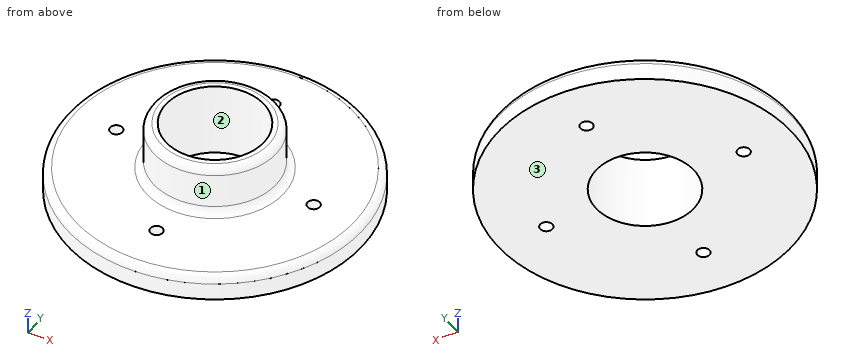
```python
from build123d import *

# Parameters (mm, degrees)
F0_R     = 76.2
F0_R_2   = 25.4
F1_DEPTH = 12.7
F2_R     = 31.75
F2_R_2   = 25.4
F3_DEPTH = 38.1
F4_R     = 3.175
F5_DEPTH = 12.701
F6_R     = 3.81


with BuildPart() as f1:
    # F0 (on Top) → F1 (new body)
    with BuildSketch(Plane.XY):
        Circle(F0_R)
        Circle(F0_R_2, mode=Mode.SUBTRACT)
    extrude(amount=F1_DEPTH)

    # F2 (on Top) → F3 (join)
    with BuildSketch(Plane.XY):
        Circle(F2_R)
        Circle(F2_R_2, mode=Mode.SUBTRACT)
    extrude(amount=F3_DEPTH)

    # F4 (on face) → F5 (cut, through all)
    with BuildSketch(Plane.XY.offset(12.7)):
        with Locations((-50.8, 0)):
            Circle(F4_R)
        with Locations((0, -50.8)):
            Circle(F4_R)
        with Locations((50.8, 0)):
            Circle(F4_R)
        with Locations((0, 50.8)):
            Circle(F4_R)
    extrude(amount=-F5_DEPTH, mode=Mode.SUBTRACT)

    # F6
    f6_edges = [f1.edges().sort_by_distance(p)[0] for p in [
        (-76.2, 0, 12.7),
        (-31.75, 0, 38.1),
        (-31.75, 0, 12.7),
    ]]
    fillet(f6_edges, radius=F6_R)


solid = f1.part
```
CAD build for the part. Positions are in the model's coordinates, mm. Face numbers are marked on the shaded views. Coordinates: 2 decimals unless noted, no trailing zeros. Write each loop counter-clockwise with the first axis right and the second up, starting at its lowest first coordinate (ties: lowest second). Pieces come first, ordered by that corner, then holes. Notation, with made-up numbers: (72, 64) -> (126, 64) arc R30 cw to (126, 86) -> close; hole circle Ø6 at (0, 80). An arc over 180 degrees is marked (long way). Return JSON: item names as keys, results as strings. Group by question number.
Q1. Cut at A-A, the plane y = 0. Give the cut face in (x, z) (3 decimals), then the cut area to 3 significant figures.
Q2. Flat gauge pins, fed straight in: pin 1 (5 mm diameter, centred on x = 14.5, z = 33, fed in from -Y); pin 2 (3 mm diameter, centred on x = -50.5, y = -45, fed in from +Z); pin 3 (2 mm diameter, centred on y = -19.5, z = 23.5, fed in from +X); pin 4 (3 mm diameter, centred on x = 53, y = -42.5, fed in from -Z). Where does each tip first touch, or does it go through?
Q3. Cut at C-C, the plane z = 5. Give the cut face in (x, y) (3 decimals), then the cut area to 3 significant figures.
Q4. Pull direction Y, two halves, no side cores. Call the marked faces 1, 2 and 3: released by +Y, released by -Y, zero draft, split by the parting line, or undercut.
Q5. Drill centre lines: line 1 (Y direction, x = 0, z = 4.5) (3 decimals); line 2 (Y direction, x = 0, z = 24); line 3 (Z direction, x = -37, y = 45). Where is each one in solid material? Low to high.
Q6. Cut at D-D, the plane z = 25.5. Give the cut face in (x, y), then the cut area to 3 significant figures.
Returned:
{
 "1": {"outline": "(-76.2, 0) -> (-53.975, 0) -> (-53.975, 12.7) -> (-72.39, 12.7) arc R3.81 ccw to (-76.2, 8.89) -> close; (-47.625, 0) -> (-25.4, 0) -> (-25.4, 38.1) -> (-27.94, 38.1) arc R3.81 ccw to (-31.75, 34.29) -> (-31.75, 16.51) arc R3.81 cw to (-35.56, 12.7) -> (-47.625, 12.7) -> close; (25.4, 0) -> (47.625, 0) -> (47.625, 12.7) -> (35.56, 12.7) arc R3.81 cw to (31.75, 16.51) -> (31.75, 34.29) arc R3.81 ccw to (27.94, 38.1) -> (25.4, 38.1) -> close; (53.975, 0) -> (76.2, 0) -> (76.2, 8.89) arc R3.81 ccw to (72.39, 12.7) -> (53.975, 12.7) -> close", "area": "1,450 mm2"},
 "2": {"pin 1": "stops at y = -29.39", "pin 2": "stops at z = 12.7", "pin 3": "stops at x = 25.8", "pin 4": "stops at z = 0"},
 "3": {"outline": "circle Ø152.4 at (0, 0); hole circle Ø6.35 at (-50.8, 0); hole circle Ø50.8 at (0, 0); hole circle Ø6.35 at (0, -50.8); hole circle Ø6.35 at (0, 50.8); hole circle Ø6.35 at (50.8, 0)", "area": "16,100 mm2"},
 "4": {"face 1": "split by the parting line", "face 2": "undercut", "face 3": "zero draft"},
 "5": {"line 1": "y = -76.2 to -53.975, -47.625 to -25.4, 25.4 to 47.625, 53.975 to 76.2", "line 2": "y = -31.75 to -25.4, 25.4 to 31.75", "line 3": "z = 0 to 12.7"},
 "6": {"outline": "circle Ø63.5 at (0, 0); hole circle Ø50.8 at (0, 0)", "area": "1,140 mm2"}
}
